Geometry: see drawing. Coordinates: mm, zero at the bounding-box minimum. Coordinates: 2 decimals unless noted, no trailing zeros. Write each loop counter-clockwise with the first axis right and the second up, starting at its lowest first coordinate (ties: lowest second). Pieces come first, ordered by that corner, then holes. Notation, with made-up numbers: M -14.5,71 L -7.5,71 A20 ccw -7.5,75 Z; hole C 75,56 d4. An arc over 180 degrees is marked long. Write item = value, one per line. Start each with the question number.
1. Section query B-B (y = 0.5). Output: boundary loops of the cut face in (x, z), then the cut area to 3 significant figures.
2. Section query C-C (z = 10.75). Output: boundary loops of the cut face in (x, y), then the cut area to 3 significant figures.
3. Section query A-A (x = 26.5). Output: boundary loops of the cut face in (y, z), then the cut area to 3 significant figures.
4. Line query: line 1 along X through (y, z) = (2.25, 9.25); line 2 along Y through (x, z) = (6.5, 5); line 3 along X through (y, z) = (0.2, 11.5). Output: solid intervals per line, ascending.
5. Pin query (flat end, axial travel): pin 1 Ø1 at (x, y) = (26.5, 2.5) entering from +Z; pin 2 Ø0.8 at (y, z) = (0.5, 11) entering from -X; pin 3 Ø6 at (x, z) = (19.5, 15) entering from -Y; pin 4 Ø1.6 at (y, z) = (2, 7.5) entering from -X. Return the tip coordinate at first contact, or that it passes through.
6. Section query D-D (x = 17.25). Output: boundary loops of the cut face in (y, z).
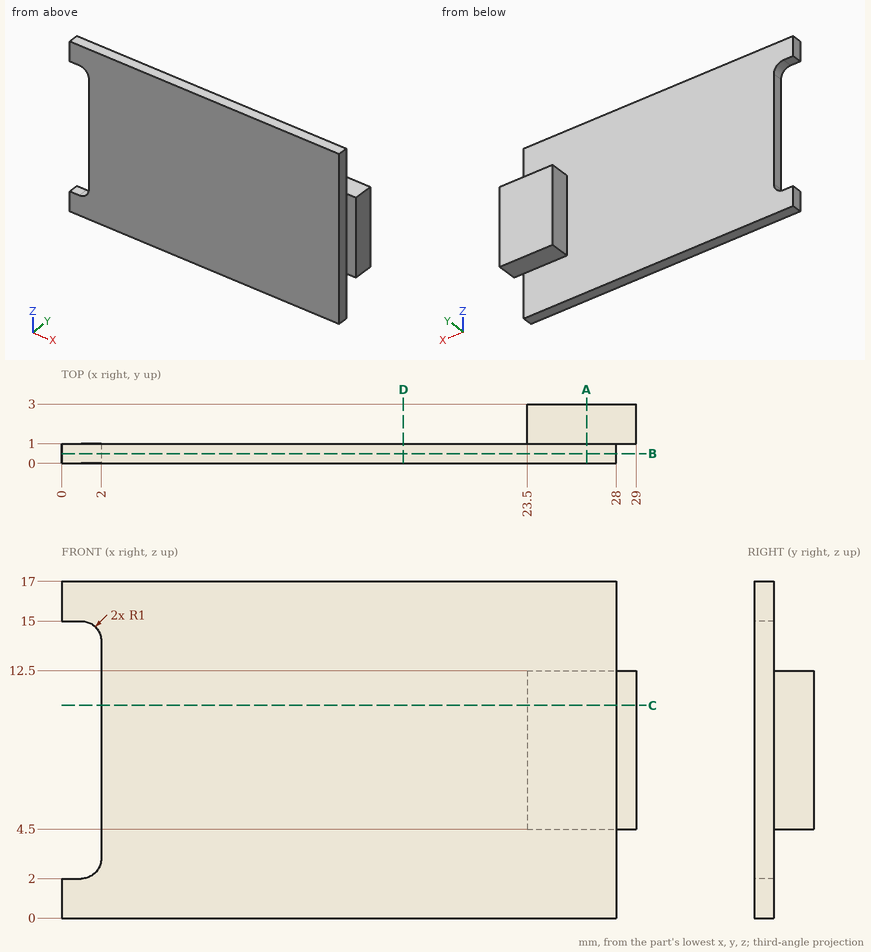
Results are:
q1.outline = M 0,0 L 28,0 L 28,17 L 0,17 L 0,15 L 1,15 A1 cw 2,14 L 2,3 A1 cw 1,2 L 0,2 Z
q1.area = 450 mm^2
q2.outline = M 2,0 L 28,0 L 28,1 L 29,1 L 29,3 L 23.5,3 L 23.5,1 L 2,1 Z
q2.area = 37.0 mm^2
q3.outline = M 0,0 L 1,0 L 1,4.5 L 3,4.5 L 3,12.5 L 1,12.5 L 1,17 L 0,17 Z
q3.area = 33.0 mm^2
q4.line_1 = 23.5 to 29
q4.line_2 = 0 to 1
q4.line_3 = 2 to 28
q5.pin_1 = 12.5
q5.pin_2 = 2
q5.pin_3 = 0
q5.pin_4 = 23.5
q6.outline = M 0,0 L 1,0 L 1,17 L 0,17 Z
